Autodesk Inventor part; units mm, degrees
ref_plane "Work Plane1" through (29, 0, 0) normal (0, -1, 0) x (1, 0, 0)
ref_plane "YZ Plane" through (0, 0, 0) normal (1, 0, 0) x (0, 1, 0)
ref_plane "XZ Plane" through (0, 0, 0) normal (0, 1, 0) x (-1, 0, 0)
sketch "Szkic1" plane through (0, 0, 0) normal (0, 0, 1) x (1, 0, 0)
  line L0 (-1.3333, 0) -> (25, 0)
  line L1 (25, 0) -> (25, 3)
  line L2 (25, 3) -> (3, 3)
  line L3 (3, 3) -> (2.3864, 3)
  line L4 (2.3864, 3) -> (0, 3)
  line L5 (0, 3) -> (0, 5)
  line L6 (0, 5) -> (-6, 5)
  line L7 (-6, 5) -> (-6, 2.8868)
  line L8 (-6, 2.8868) -> (-3, 2.8868)
  line L9 (-3, 2.8868) -> (-1.3333, 0)
  line L10 (-12.2, 0) -> (31.2, 0)
  line L11 (0, -1) -> (0, 6)
  line L12 (3, 3) -> (0, 3) construction
  dimension "d1" = 22
  dimension "d2" = 0.6136
  dimension "d3" = 6
  dimension "d4" = 3
  dimension "d5" = 60
  dimension "d6" = 6
  dimension "d7" = 6
  dimension "d8" = 5.7735
  dimension "d9" = 10
  dimension "d26" = 25
revolve "Bryła" add sketch "Szkic1" angle 360 about axis through (-1.3333, 0, 0) along (1, 0, 0)
sketch "Szkic2" plane through (-6, 0, 0) normal (-1, 0, 0) x (0, 0, 1)
  circle A0 centre (0, 0) radius 2.8868
  line L0 (0, -7) -> (0, 7)
  line L1 (-7, 0) -> (7, 0)
  line L2 (2.8868, 0) -> (1.4434, -2.5)
  line L3 (1.4434, -2.5) -> (-1.4434, -2.5)
  line L4 (-1.4434, -2.5) -> (-2.8868, 0)
  line L5 (-2.8868, 0) -> (-1.4434, 2.5)
  line L6 (-1.4434, 2.5) -> (1.4434, 2.5)
  line L7 (1.4434, 2.5) -> (2.8868, 0)
extrude "Szczelina" add sketch "Szkic2" against normal up to next contours L7 A0 | A0 L2 | L6 L0 A0 | A0 L0 L3 | L0 L6 A0 | A0 L3 L0 | L4 A0 | A0 L5
fillet "Zaokrąglenie1" radius 0.6 1 edges at (-6, -5, 0)
thread "Gwint"
chamfer "Faza1" distance 0.6135 distance2 0.6135 1 edges at (25, -3, 0) measured on face at (25, -0.5681, -0.823)
ref_plane "Work Plane1" through (29, 0, 0) normal (0, -1, 0) x (1, 0, 0)
fillet "Fillet2" radius 0.1 1 edges at (0, -3, 0)
equation "\"d1\" = GEL"
equation "\"d3\" = KOH"
equation "\"d4\" = INTI"
equation "\"d6\" = GD"
equation "\"d7\" = BDM"
equation "\"d8\" = 1.1547 * SW"
equation "\"d9\" = KOD"
equation "\"d26\" = NLG"
equation "\"d30\" = R"
equation "\"d17\" = RR"
equation "\"d13\" = GEL"
equation "\"d15\" = -0.5 * SPD + 0.5 * GD"
equation "\"d16\" = GUL"
equation "\"GD\" = 6"
equation "\"NLG\" = 25"
equation "\"GEL\" = 22"
equation "\"KOD\" = 10"
equation "\"KOH\" = 6"
equation "\"INTI\" = 3"
equation "\"GAL\" = 0.61345 * PTC"
equation "\"GUL\" = 0.61345 * PTC"
equation "\"BDM\" = NND"
equation "\"SW\" = 5"
equation "\"RR\" = 0.6"
equation "\"SPD\" = NND - 1.2269 * PTC"
equation "\"R\" = 0.1"
equation "\"TOA\" = 30deg"
equation "\"GD1\" = THREADDIA - 1.2269 * PTC"
equation "\"THREADDIA\" = 6"
equation "\"FAWI\" = 45deg"
equation "\"PTC\" = 1"
equation "\"NND\" = 6"
equation "\"E0\" = 1.155 * SW"
properties part number "ISO 4762  - M6 x 25" material "Stal nierdzewna 440C"
Could you check a few things on this model? Use its own coordinates, in mm. A direction names the side the tool comes from. Give positions to 0.01 mm unless a question says otherwise; leave off trailing zeros. Write each loop counter-clockwise with the first axis right and the second up, starting at its lowest first coordinate (ties: lowest second). Pieces come first, ordered by that corner, then holes. Notation, with made-up numbers: (36, -13) -> (64, -13) arc R17 cw to (64, 18) -> close; hole circle Ø11 at (-18, 13). An arc over 180 degrees is marked (long way). Write each question's results on one line, items separated by ' | '. Start each with the question number.
Q1. I'm going to push flat-ended pins straight in: pin 1 Ø2 at (y, z) = (3, 2.5) entering from +X; pin 2 Ø6 at (x, y) = (7.5, -1) entering from +Z; pin 3 Ø6 at (x, z) = (12.5, 3) entering from -Y. Where does each tip first touch, or does it pass through?
Q2. We'd pull the mould along Y, two halves only. Please class faces 1 (the face through (25, 0, 0)), 2 (the face through (-4, 2.5, 0)), 3 (the face through (-2.74, -1.08, 4.88)): +Y half, -Y half, draft (parallel to the pull), parting line (faces both ways), or undercut.
Q3. Suppose I cut it at A-A, the plane x = 5. List the corners of the cut face in (y, z) for me, and give its area (3 significant figures).
Q4. Which directions (+Z, -Z, +X, -X, +Y, -Y) give clear straight access to the entire face, cutting with the end or side of a thin tool? Please do faces 4 (the face through (12, -3, 0)), 5 (the face through (-4.411, 1.268, 2.155)), 6 (the face through (-6, -2, 2)).
Q5. I need wall thicknesses on probe 1 along X at (y, z) = (-2, 3.25); probe 2 along Z at (x, y) = (-2, -0.25); probe 3 along Y at (x, z) = (22.5, -1.75). Which ranges of each line are inside material? Lowest first, please.
Outcome:
1) pin 1: x = 24.48 | pin 2: z = 3 | pin 3: y = -3
2) face 1: draft | face 2: undercut | face 3: parting line
3) outline: circle Ø6 at (0, 0) | area: 28.3 mm2
4) face 4: +X | face 5: -X | face 6: +Z, -Z, -X, +Y, -Y
5) probe 1: -6 to 0 | probe 2: -4.99 to -1.13, 1.13 to 4.99 | probe 3: -2.44 to 2.44
